Design review of the part shown in the three views and the two pictorial views. Dimensions are in mm from the part's minimum x, y and z. A direction names the side the tool comes from. Coordinates: 2 decimals unless noted, no trailing zeros. Loops run counter-clockwise (first coordinate to the right, second up) from the corner with the lowest first, then second, coordinate; pieces in that order, holes last. Notation, with made-up numbers: (88, -38) - (99, -38) arc R31 cw to (99, -11) - close; hole circle Ø6 at (-37, 15). An arc over 180 degrees is marked (long way). One line per item, written item: value. Start each with the question number.
1. The part is to be moulded in two halves that separate along X. For the marked faces 6, 7 and 8, say which applies: released by +X, released by -X, zero draft, split by the parting line, or undercut.
2. Take a section at A-A, the plane y = 8. State the section outline as (x, z) points.
3. For the marked faces 1, 2, 3, 4 and 5, list the 3-axis set-ups (+Z, -Z, +X, -X, +Y, -Y) from which the entire face can be reached by the end or side of a thin tool; tool diameter is ignored.
4. Insertion check: pin 1 (3 mm diameter, centred on y = 5.5, z = 6.5, fed in from +X); pin 2 (6 mm diameter, centred on x = 48, z = 31, fed in from -Y); pin 3 (13.5 mm diameter, centred on x = 27.5, z = 45, fed in from +Y); pin 4 (2 mm diameter, centred on x = 17, z = 35.5, fed in from +Y). Each pin has a flat end and moves straight along its axis. Give the tip position at first contact, or say it passes through.
5. To check wall thickness, follow line 1 (X direction, y = 24.5, z = 45); line 2 (Z direction, x = 26, y = 9.5); line 3 (Z direction, x = 27, y = 25). State the ranges of each line that lie inside material, in increasing order. Write a range as from..to.
6. Take a section at D-D, the plane z = 45. State the section outline as (x, y) points.
7. Take a section at B-B, the plane x = 27.5. State the section outline as (y, z) points, and give its area (3 significant figures).
8. Take a section at C-C, the plane y = 34. State the section outline as (x, z) points.
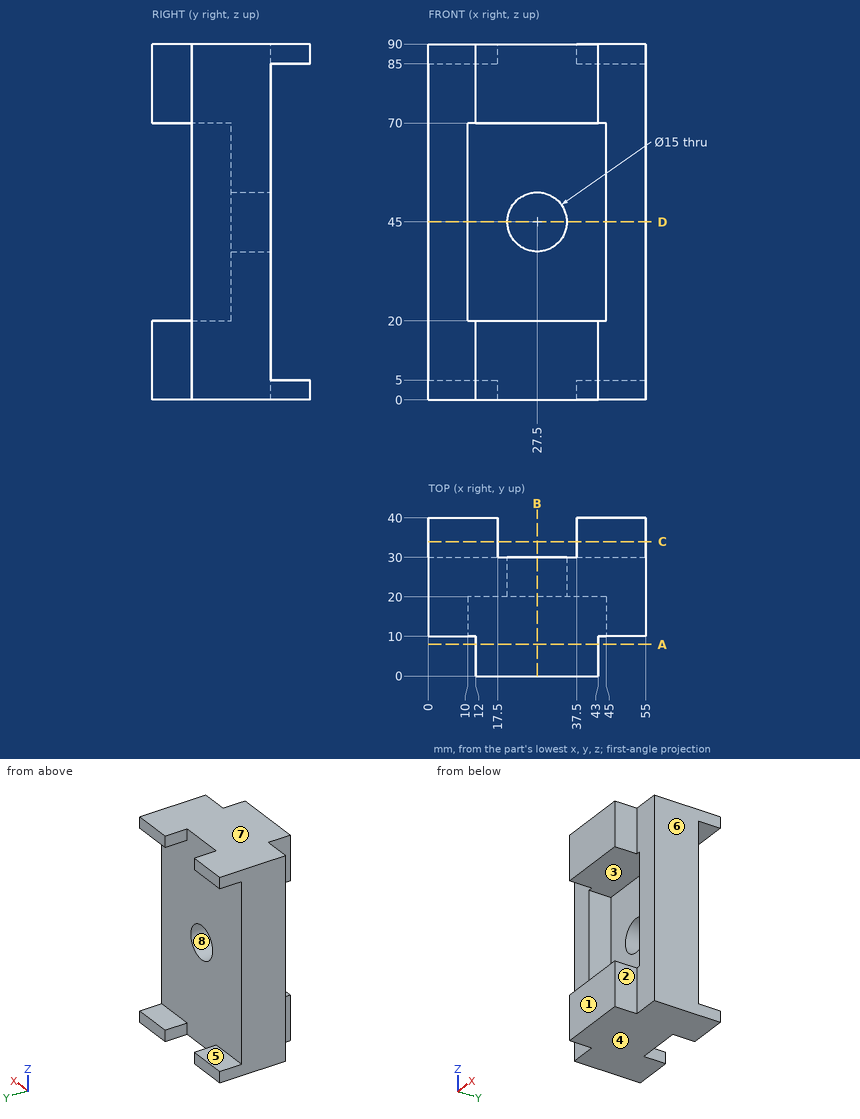
Solutions:
1. face 6: released by +X
1. face 7: zero draft
1. face 8: undercut
2. outline: (12, 0) - (43, 0) - (43, 20) - (12, 20) - close; (12, 70) - (43, 70) - (43, 90) - (12, 90) - close
3. face 1: +Z, -Z, +X, -X, -Y
3. face 2: +Z, -Z, +X, -Y
3. face 3: -Y
3. face 4: -Z, +X, -X, +Y, -Y
3. face 5: +X, -X, +Y
4. pin 1: x = 43
4. pin 2: y = 10
4. pin 3: through
4. pin 4: y = 30
5. line 1: 0..20, 35..55
5. line 2: 0..20, 70..90
5. line 3: 0..37.52, 52.48..90
6. outline: (0, 10) - (10, 10) - (10, 20) - (20, 20) - (20, 30) - (0, 30) - close; (35, 20) - (45, 20) - (45, 10) - (55, 10) - (55, 30) - (35, 30) - close
7. outline: (0, 0) - (30, 0) - (30, 37.5) - (20, 37.5) - (20, 20) - (0, 20) - close; (0, 70) - (20, 70) - (20, 52.5) - (30, 52.5) - (30, 90) - (0, 90) - close
7. area: 1,550 mm2
8. outline: (0, 0) - (17.5, 0) - (17.5, 5) - (0, 5) - close; (0, 85) - (17.5, 85) - (17.5, 90) - (0, 90) - close; (37.5, 0) - (55, 0) - (55, 5) - (37.5, 5) - close; (37.5, 85) - (55, 85) - (55, 90) - (37.5, 90) - close
